from build123d import *

# Parameters (mm, degrees)
BOSS_EXTRUDE1_DEPTH = 2
SKETCH8_R           = 1.1
BOSS_EXTRUDE4_DEPTH = 5
SKETCH2_W           = 75
SKETCH2_H           = 2
BOSS_EXTRUDE2_DEPTH = 65
SKETCH9_W           = 15
SKETCH9_H           = 20
CUT_EXTRUDE2_DEPTH  = 120.921849552
SKETCH10_R          = 1.375
CUT_EXTRUDE3_DEPTH  = 122.017560709
SKETCH11_R          = 3
SKETCH11_R_2        = 1.375
BOSS_EXTRUDE5_DEPTH = 2
CUT_EXTRUDE4_DEPTH  = 121.371300566
SKETCH16_W          = 5.5
SKETCH16_H          = 5
CUT_EXTRUDE5_DEPTH  = 118.032046893
SKETCH17_W          = 6
SKETCH17_H          = 38
BOSS_EXTRUDE6_DEPTH = 3
SKETCH18_W          = 51
SKETCH18_H          = 13
CUT_EXTRUDE6_DEPTH  = 118.032046893
FILLET1_R           = 1


with BuildPart() as part:
    # Sketch1 → Boss-Extrude1 (new body)
    with BuildSketch(Plane.XY):
        Polygon((-50, 5), (-50, 0), (25, 0), (25, 5), (92.5, 5), (92.5, 40), (57.5, 40), (-57.5, 40), (-92.5, 40), (-92.5, 5), align=None)
    extrude(amount=BOSS_EXTRUDE1_DEPTH)

    # Sketch8 → Boss-Extrude4 (add)
    with BuildSketch(Plane.XY.offset(2)):
        with Locations((-85.5, 33)):
            Circle(SKETCH8_R)
        with Locations((-64.5, 33)):
            Circle(SKETCH8_R)
        with Locations((-85.5, 20.5)):
            Circle(SKETCH8_R)
        with Locations((-64.5, 20.5)):
            Circle(SKETCH8_R)
    boss_extrude4 = extrude(amount=BOSS_EXTRUDE4_DEPTH)

    # Mirror2: Boss-Extrude4 across plane
    add(boss_extrude4.mirror(Plane(origin=(0, 0, 0), x_dir=(0, 0, 1), z_dir=(1, 0, 0))))

    # Sketch2 → Boss-Extrude2 (add)
    with BuildSketch(Plane.XY.offset(2)):
        with Locations((-12.5, 1)):
            Rectangle(SKETCH2_W, SKETCH2_H)
    extrude(amount=BOSS_EXTRUDE2_DEPTH)

    # Sketch9 → Cut-Extrude2 (cut, through all)
    with BuildSketch(Plane.XY.offset(2)):
        with Locations((-75, 23.069)):
            Rectangle(SKETCH9_W, SKETCH9_H)
        with Locations((75, 23.069)):
            Rectangle(SKETCH9_W, SKETCH9_H)
    extrude(amount=-CUT_EXTRUDE2_DEPTH, mode=Mode.SUBTRACT)

    # Sketch10 → Cut-Extrude3 (cut, through all)
    with BuildSketch(Plane.XZ):
        with Locations(Location((-41.5, 58.5, 0), (0, 0, 270))):
            Circle(SKETCH10_R)
        with Locations(Location((-41.5, 9.5, 0), (0, 0, 270))):
            Circle(SKETCH10_R)
        with Locations(Location((16.5, 9.5, 0), (0, 0, 270))):
            Circle(SKETCH10_R)
        with Locations(Location((16.5, 58.5, 0), (0, 0, 270))):
            Circle(SKETCH10_R)
    extrude(amount=-CUT_EXTRUDE3_DEPTH, mode=Mode.SUBTRACT)

    # Sketch11 → Boss-Extrude5 (add)
    with BuildSketch(Plane(origin=(0, 2, 0), x_dir=(1, 0, 0), z_dir=(0, 1, 0))):
        with Locations((-41.5, -9.5)):
            Circle(SKETCH11_R)
        with Locations(Location((-41.5, -9.5, 0), (0, 0, 90))):
            Circle(SKETCH11_R_2, mode=Mode.SUBTRACT)
    boss_extrude5 = extrude(amount=BOSS_EXTRUDE5_DEPTH)

    # Sketch-Pattern1: Boss-Extrude5 at 3 more places
    with Locations((58, 0, 0), (58, 0, 49), (0, 0, 49)):
        add(boss_extrude5)

    # Sketch15 → Cut-Extrude4 (cut, through all)
    with BuildSketch(Plane(origin=(0, 2, 0), x_dir=(1, 0, 0), z_dir=(0, 1, 0))):
        with BuildLine():
            ThreePointArc((-42.7, -12.249545417), (-44.00998008, -11.143167673), (-44.5, -9.5))
            Line((-44.5, -9.5), (-44.5, -2))
            Line((-44.5, -2), (-50, -2))
            Line((-50, -2), (-50, -67))
            Line((-50, -67), (25, -67))
            Line((25, -67), (25, -2))
            Line((25, -2), (19.5, -2))
            Line((19.5, -2), (19.5, -9.5))
            ThreePointArc((19.5, -9.5), (19.00998008, -11.143167673), (17.7, -12.249545417))
            ThreePointArc((17.7, -12.249545417), (16.826679947, -12.98713058), (16.5, -14.082575695))
            Line((16.5, -14.082575695), (16.5, -53.428932188))
            ThreePointArc((16.5, -53.428932188), (16.652240935, -54.194299053), (17.085786438, -54.843145751))
            Line((17.085786438, -54.843145751), (18.621320344, -56.378679656))
            ThreePointArc((18.621320344, -56.378679656), (19.271638598, -57.351949703), (19.5, -58.5))
            ThreePointArc((19.5, -58.5), (17.648050297, -61.271638598), (14.378679656, -60.621320344))
            Line((14.378679656, -60.621320344), (12.843145751, -59.085786438))
            ThreePointArc((12.843145751, -59.085786438), (12.194299053, -58.652240935), (11.428932188, -58.5))
            Line((11.428932188, -58.5), (-36.428932188, -58.5))
            ThreePointArc((-36.428932188, -58.5), (-37.194299053, -58.652240935), (-37.843145751, -59.085786438))
            Line((-37.843145751, -59.085786438), (-39.378679656, -60.621320344))
            ThreePointArc((-39.378679656, -60.621320344), (-43.621320344, -60.621320344), (-43.621320344, -56.378679656))
            Line((-43.621320344, -56.378679656), (-42.085786438, -54.843145751))
            ThreePointArc((-42.085786438, -54.843145751), (-41.652240935, -54.194299053), (-41.5, -53.428932188))
            Line((-41.5, -53.428932188), (-41.5, -14.082575695))
            ThreePointArc((-41.5, -14.082575695), (-41.826679947, -12.98713058), (-42.7, -12.249545417))
        make_face()
    extrude(amount=-CUT_EXTRUDE4_DEPTH, mode=Mode.SUBTRACT)

    # Sketch16 → Cut-Extrude5 (cut, through all)
    with BuildSketch(Plane.XY.offset(2)):
        with Locations((-47.25, 2.5)):
            Rectangle(SKETCH16_W, SKETCH16_H)
        with Locations((22.25, 2.5)):
            Rectangle(SKETCH16_W, SKETCH16_H)
    extrude(amount=-CUT_EXTRUDE5_DEPTH, mode=Mode.SUBTRACT)

    # Sketch17 → Boss-Extrude6 (add)
    with BuildSketch(Plane.XY.offset(2)):
        with Locations((-41.5, 21)):
            Rectangle(SKETCH17_W, SKETCH17_H)
        with Locations((16.5, 21)):
            Rectangle(SKETCH17_W, SKETCH17_H)
    extrude(amount=BOSS_EXTRUDE6_DEPTH)

    # Sketch18 → Cut-Extrude6 (cut, through all)
    with BuildSketch(Plane.XY.offset(2)):
        with Locations((-12.5, 13.5)):
            Rectangle(SKETCH18_W, SKETCH18_H)
    extrude(amount=-CUT_EXTRUDE6_DEPTH, mode=Mode.SUBTRACT)

    # Fillet1
    fillet1_edges = [part.edges().sort_by_distance(p)[0] for p in [
        (-38, 20, 1),
        (13, 20, 1),
        (13, 7, 1),
        (-38, 7, 1),
    ]]
    fillet(fillet1_edges, radius=FILLET1_R)


solid = part.part
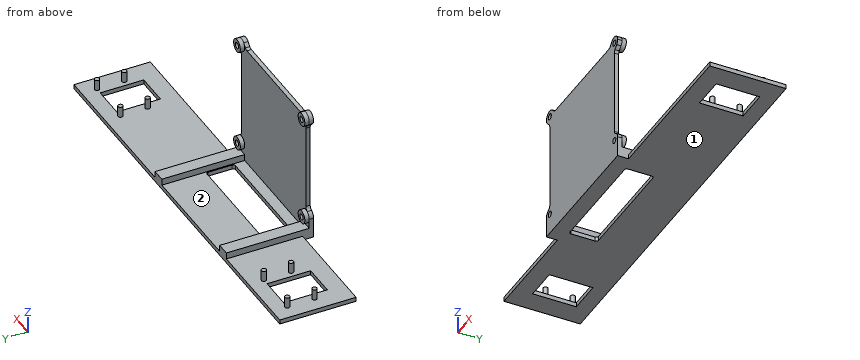
For this review, take the finished solid that the model builds, in its own axes (mm). Face numbers are marked on the shaded views. A direction names the side the tool comes from. Coordinates: 2 decimals unless noted, no trailing zeros. Loops run counter-clockwise (first coordinate to the right, second up) from the corner with the lowest first, then second, coordinate; pieces in that order, holes last. Notation, with made-up numbers: (-20.75, -16.5) - (34.25, -16.5) arc R17 cw to (34.25, 7.5) - close; hole circle Ø10 at (16.25, 32). An arc over 180 degrees is marked (long way). Use a Markdown table: item, result. Add a question column.
Item 1: We need section A-A (y = 11). Give the boundary of the cut face in (x, z).
Item 2: For line 1 (X direction, y = 3.45, z = 58.5) (3 decimals); line 2 (Z direction, x = -41.5, y = 3) (3 decimals); line 3 (X direction, y = 36, z = 3), list the stretches that pass through material, from the lowest coordinate up.
Item 3: We need section B-B (z = 20). Give the boundary of the cut face in (x, y), and give its area (3 significant figures).
Item 4: Insertion check: pin 1 Ø2.5 at (x, y) = (65, 33) entering from +Z; pin 2 Ø2.5 at (x, z) = (-41.5, 58.5) entering from -Y; pin 3 Ø1.6 at (x, z) = (73, 1) entering from -Y; pin 4 Ø8 at (x, y) = (-6.5, 19) entering from +Z. Each pin has a flat end and moves straight along its axis. Give the tip position at first contact, or say it passes through.
Item 5: We need section C-C (x = -59). Give the boundary of the cut face in (y, z), and give its area (3 significant figures).
Item 6: Tool access review of the marked faces 1 and 2: name each direction out of +Z, -Z, +X, -X, +Y, -Y from which nothing blocks a thin tool from reaching the whole face with its end or side.
Results list:
| question | item | result |
|---|---|---|
| 1 | outline | (-92.5, 0) - (-38, 0) - (-38, 2) - (-38.5, 2) - (-38.5, 5) - (-44.5, 5) - (-44.5, 2) - (-92.5, 2) - close; (13, 0) - (92.5, 0) - (92.5, 2) - (19.5, 2) - (19.5, 5) - (13.5, 5) - (13.5, 2) - (13, 2) - close |
| 2 | line 1 | x = -44.5 to -42.875, -40.125 to -38.5, 13.5 to 15.125, 17.875 to 19.5 |
| 2 | line 2 | z = 0 to 5, 6.5 to 8.125, 10.875 to 12.5, 55.5 to 57.125, 59.875 to 61.5 |
| 2 | line 3 | x = -44.5 to -38.5, 13.5 to 19.5 |
| 3 | outline | (-41.5, 0) - (16.5, 0) - (16.5, 2) - (-41.5, 2) - close |
| 3 | area | 116 mm^2 |
| 4 | pin 1 | stops at z = 7 |
| 4 | pin 2 | passes through |
| 4 | pin 3 | stops at y = 5 |
| 4 | pin 4 | stops at z = 2 |
| 5 | outline | (5, 0) - (40, 0) - (40, 2) - (5, 2) - close |
| 5 | area | 70.0 mm^2 |
| 6 | face 1 | -Z, +X, -X, +Y, -Y |
| 6 | face 2 | +Z, +Y |
